Verification items for the finished model (mm, model axes). A direction names the side the tool comes from. Coordinates: 2 decimals unless noted, no trailing zeros. Write each loop counter-clockwise with the first axis right and the second up, starting at its lowest first coordinate (ties: lowest second). Pieces come first, ordered by that corner, then holes. Notation, with made-up numbers: (0.5, -18) -> (57.5, -18) arc R9 ccw to (57.5, -8) -> close; hole circle Ø9 at (-3, 40.5). An arc over 180 degrees is marked (long way). Answer in a Markdown table with one row per item.
```python
from build123d import *

# Parameters (mm, degrees)
SKETCH1_R           = 11
BOSS_EXTRUDE1_DEPTH = 5
BOSS_EXTRUDE2_START = -4
BOSS_EXTRUDE2_DEPTH = 2.5


with BuildPart() as part:
    # Sketch1 → Boss-Extrude1 (new body)
    with BuildSketch(Plane.XY):
        with BuildLine():
            ThreePointArc((4, -41.6), (7.535533906, -43.064466094), (9, -46.6))
            Line((9, -46.6), (9, -61.492137976))
            ThreePointArc((9, -61.492137976), (20.215230476, -65.413125036), (26.544375, -75.467848491))
            ThreePointArc((26.544375, -75.467848491), (30.614674589, -73.910362601), (34.594119865, -72.133534994))
            ThreePointArc((34.594119865, -72.133534994), (31.959737739, -60.548390845), (37.117546722, -49.845468783))
            Line((37.117546722, -49.845468783), (26.587214973, -39.315137034))
            ThreePointArc((26.587214973, -39.315137034), (25.122748879, -35.779603128), (26.587214973, -32.244069222))
            Line((26.587214973, -32.244069222), (32.244069222, -26.587214973))
            ThreePointArc((32.244069222, -26.587214973), (35.779603128, -25.122748879), (39.315137034, -26.587214973))
            Line((39.315137034, -26.587214973), (49.845468783, -37.117546722))
            ThreePointArc((49.845468783, -37.117546722), (60.548390845, -31.959737739), (72.133534994, -34.594119865))
            ThreePointArc((72.133534994, -34.594119865), (73.910362601, -30.614674589), (75.467848491, -26.544375))
            ThreePointArc((75.467848491, -26.544375), (65.413125036, -20.215230476), (61.492137976, -9))
            Line((61.492137976, -9), (46.6, -9))
            ThreePointArc((46.6, -9), (43.064466094, -7.535533906), (41.6, -4))
            Line((41.6, -4), (41.6, 4))
            ThreePointArc((41.6, 4), (43.064466094, 7.535533906), (46.6, 9))
            Line((46.6, 9), (61.492137976, 9))
            ThreePointArc((61.492137976, 9), (65.413125036, 20.215230476), (75.467848491, 26.544375))
            ThreePointArc((75.467848491, 26.544375), (73.910362601, 30.614674589), (72.133534994, 34.594119865))
            ThreePointArc((72.133534994, 34.594119865), (60.548390845, 31.959737739), (49.845468783, 37.117546722))
            Line((49.845468783, 37.117546722), (39.315137034, 26.587214973))
            ThreePointArc((39.315137034, 26.587214973), (35.779603128, 25.122748879), (32.244069222, 26.587214973))
            Line((32.244069222, 26.587214973), (26.587214973, 32.244069222))
            ThreePointArc((26.587214973, 32.244069222), (25.122748879, 35.779603128), (26.587214973, 39.315137034))
            Line((26.587214973, 39.315137034), (37.117546722, 49.845468783))
            ThreePointArc((37.117546722, 49.845468783), (31.959737739, 60.548390845), (34.594119865, 72.133534994))
            ThreePointArc((34.594119865, 72.133534994), (30.614674589, 73.910362601), (26.544375, 75.467848491))
            ThreePointArc((26.544375, 75.467848491), (20.215230476, 65.413125036), (9, 61.492137976))
            Line((9, 61.492137976), (9, 46.6))
            ThreePointArc((9, 46.6), (7.535533906, 43.064466094), (4, 41.6))
            Line((4, 41.6), (-4, 41.6))
            ThreePointArc((-4, 41.6), (-7.535533906, 43.064466094), (-9, 46.6))
            Line((-9, 46.6), (-9, 61.492137976))
            ThreePointArc((-9, 61.492137976), (-20.215230476, 65.413125036), (-26.544375, 75.467848491))
            ThreePointArc((-26.544375, 75.467848491), (-30.614674589, 73.910362601), (-34.594119865, 72.133534994))
            ThreePointArc((-34.594119865, 72.133534994), (-31.959737739, 60.548390845), (-37.117546722, 49.845468783))
            Line((-37.117546722, 49.845468783), (-26.587214973, 39.315137034))
            ThreePointArc((-26.587214973, 39.315137034), (-25.122748879, 35.779603128), (-26.587214973, 32.244069222))
            Line((-26.587214973, 32.244069222), (-32.244069222, 26.587214973))
            ThreePointArc((-32.244069222, 26.587214973), (-35.779603128, 25.122748879), (-39.315137034, 26.587214973))
            Line((-39.315137034, 26.587214973), (-49.845468783, 37.117546722))
            ThreePointArc((-49.845468783, 37.117546722), (-60.548390845, 31.959737739), (-72.133534994, 34.594119865))
            ThreePointArc((-72.133534994, 34.594119865), (-73.910362601, 30.614674589), (-75.467848491, 26.544375))
            ThreePointArc((-75.467848491, 26.544375), (-65.413125036, 20.215230476), (-61.492137976, 9))
            Line((-61.492137976, 9), (-46.6, 9))
            ThreePointArc((-46.6, 9), (-43.064466094, 7.535533906), (-41.6, 4))
            Line((-41.6, 4), (-41.6, -4))
            ThreePointArc((-41.6, -4), (-43.064466094, -7.535533906), (-46.6, -9))
            Line((-46.6, -9), (-61.492137976, -9))
            ThreePointArc((-61.492137976, -9), (-65.413125036, -20.215230476), (-75.467848491, -26.544375))
            ThreePointArc((-75.467848491, -26.544375), (-73.910362601, -30.614674589), (-72.133534994, -34.594119865))
            ThreePointArc((-72.133534994, -34.594119865), (-60.548390845, -31.959737739), (-49.845468783, -37.117546722))
            Line((-49.845468783, -37.117546722), (-39.315137034, -26.587214973))
            ThreePointArc((-39.315137034, -26.587214973), (-35.779603128, -25.122748879), (-32.244069222, -26.587214973))
            Line((-32.244069222, -26.587214973), (-26.587214973, -32.244069222))
            ThreePointArc((-26.587214973, -32.244069222), (-25.122748879, -35.779603128), (-26.587214973, -39.315137034))
            Line((-26.587214973, -39.315137034), (-37.117546722, -49.845468783))
            ThreePointArc((-37.117546722, -49.845468783), (-31.959737739, -60.548390845), (-34.594119865, -72.133534994))
            ThreePointArc((-34.594119865, -72.133534994), (-30.614674589, -73.910362601), (-26.544375, -75.467848491))
            ThreePointArc((-26.544375, -75.467848491), (-20.215230476, -65.413125036), (-9, -61.492137976))
            Line((-9, -61.492137976), (-9, -46.6))
            ThreePointArc((-9, -46.6), (-7.535533906, -43.064466094), (-4, -41.6))
            Line((-4, -41.6), (4, -41.6))
        make_face()
        Circle(SKETCH1_R, mode=Mode.SUBTRACT)
    extrude(amount=BOSS_EXTRUDE1_DEPTH)

    # Sketch2 → Boss-Extrude2 (add)
    with BuildSketch(Plane.XY.offset(5).offset(BOSS_EXTRUDE2_START)):
        with BuildLine():
            ThreePointArc((-37.117546722, 49.845468783), (-31.959737739, 60.548390845), (-34.594119865, 72.133534994))
            ThreePointArc((-34.594119865, 72.133534994), (-42.489529555, 67.783772971), (-49.845468783, 62.573390845))
            Line((-49.845468783, 62.573390845), (-37.117546722, 49.845468783))
        make_face()
        with BuildLine():
            Line((-49.845468783, 37.117546722), (-62.573390845, 49.845468783))
            ThreePointArc((-62.573390845, 49.845468783), (-67.783772971, 42.489529555), (-72.133534994, 34.594119865))
            ThreePointArc((-72.133534994, 34.594119865), (-60.548390845, 31.959737739), (-49.845468783, 37.117546722))
        make_face()
        with BuildLine():
            Line((-9, 61.492137976), (-9, 79.492137976))
            ThreePointArc((-9, 79.492137976), (-17.885731045, 77.975), (-26.544375, 75.467848491))
            ThreePointArc((-26.544375, 75.467848491), (-20.215230476, 65.413125036), (-9, 61.492137976))
        make_face()
        with BuildLine():
            ThreePointArc((9, 61.492137976), (20.215230476, 65.413125036), (26.544375, 75.467848491))
            ThreePointArc((26.544375, 75.467848491), (17.885731045, 77.975), (9, 79.492137976))
            Line((9, 79.492137976), (9, 61.492137976))
        make_face()
        with BuildLine():
            Line((37.117546722, 49.845468783), (49.845468783, 62.573390845))
            ThreePointArc((49.845468783, 62.573390845), (42.489529555, 67.783772971), (34.594119865, 72.133534994))
            ThreePointArc((34.594119865, 72.133534994), (31.959737739, 60.548390845), (37.117546722, 49.845468783))
        make_face()
        with BuildLine():
            ThreePointArc((49.845468783, 37.117546722), (60.548390845, 31.959737739), (72.133534994, 34.594119865))
            ThreePointArc((72.133534994, 34.594119865), (67.783772971, 42.489529555), (62.573390845, 49.845468783))
            Line((62.573390845, 49.845468783), (49.845468783, 37.117546722))
        make_face()
        with BuildLine():
            Line((61.492137976, 9), (79.492137976, 9))
            ThreePointArc((79.492137976, 9), (77.975, 17.885731045), (75.467848491, 26.544375))
            ThreePointArc((75.467848491, 26.544375), (65.413125036, 20.215230476), (61.492137976, 9))
        make_face()
        with BuildLine():
            Line((79.492137976, -9), (61.492137976, -9))
            ThreePointArc((61.492137976, -9), (65.413125036, -20.215230476), (75.467848491, -26.544375))
            ThreePointArc((75.467848491, -26.544375), (77.975, -17.885731045), (79.492137976, -9))
        make_face()
        with BuildLine():
            ThreePointArc((62.573390845, -49.845468783), (67.783772971, -42.489529555), (72.133534994, -34.594119865))
            ThreePointArc((72.133534994, -34.594119865), (60.548390845, -31.959737739), (49.845468783, -37.117546722))
            Line((49.845468783, -37.117546722), (62.573390845, -49.845468783))
        make_face()
        with BuildLine():
            ThreePointArc((34.594119865, -72.133534994), (42.489529555, -67.783772971), (49.845468783, -62.573390845))
            Line((49.845468783, -62.573390845), (37.117546722, -49.845468783))
            ThreePointArc((37.117546722, -49.845468783), (31.959737739, -60.548390845), (34.594119865, -72.133534994))
        make_face()
        with BuildLine():
            ThreePointArc((9, -79.492137976), (17.885731045, -77.975), (26.544375, -75.467848491))
            ThreePointArc((26.544375, -75.467848491), (20.215230476, -65.413125036), (9, -61.492137976))
            Line((9, -61.492137976), (9, -79.492137976))
        make_face()
        with BuildLine():
            ThreePointArc((-26.544375, -75.467848491), (-17.885731045, -77.975), (-9, -79.492137976))
            Line((-9, -79.492137976), (-9, -61.492137976))
            ThreePointArc((-9, -61.492137976), (-20.215230476, -65.413125036), (-26.544375, -75.467848491))
        make_face()
        with BuildLine():
            ThreePointArc((-49.845468783, -62.573390845), (-42.489529555, -67.783772971), (-34.594119865, -72.133534994))
            ThreePointArc((-34.594119865, -72.133534994), (-31.959737739, -60.548390845), (-37.117546722, -49.845468783))
            Line((-37.117546722, -49.845468783), (-49.845468783, -62.573390845))
        make_face()
        with BuildLine():
            ThreePointArc((-72.133534994, -34.594119865), (-67.783772971, -42.489529555), (-62.573390845, -49.845468783))
            Line((-62.573390845, -49.845468783), (-49.845468783, -37.117546722))
            ThreePointArc((-49.845468783, -37.117546722), (-60.548390845, -31.959737739), (-72.133534994, -34.594119865))
        make_face()
        with BuildLine():
            ThreePointArc((-79.492137976, -9), (-77.975, -17.885731045), (-75.467848491, -26.544375))
            ThreePointArc((-75.467848491, -26.544375), (-65.413125036, -20.215230476), (-61.492137976, -9))
            Line((-61.492137976, -9), (-79.492137976, -9))
        make_face()
        with BuildLine():
            ThreePointArc((-75.467848491, 26.544375), (-77.975, 17.885731045), (-79.492137976, 9))
            Line((-79.492137976, 9), (-61.492137976, 9))
            ThreePointArc((-61.492137976, 9), (-65.413125036, 20.215230476), (-75.467848491, 26.544375))
        make_face()
    extrude(amount=BOSS_EXTRUDE2_DEPTH)


solid = part.part
```
1. Sectioned sample at D-D, the plane x = 69.5. Record the cut outline in (y, z).
Findings below:
| item | result |
|---|---|
| outline | (-39.62, 1) -> (-33.23, 1) -> (-33.23, 0) -> (-23.97, 0) -> (-23.97, 1) -> (-9, 1) -> (-9, 3.5) -> (-23.97, 3.5) -> (-23.97, 5) -> (-33.23, 5) -> (-33.23, 3.5) -> (-39.62, 3.5) -> close; (9, 1) -> (23.97, 1) -> (23.97, 0) -> (33.23, 0) -> (33.23, 1) -> (39.62, 1) -> (39.62, 3.5) -> (33.23, 3.5) -> (33.23, 5) -> (23.97, 5) -> (23.97, 3.5) -> (9, 3.5) -> close |
2. Access from +Z, -Z, +X, -X, +Y, -Y to the whole of each face (thin tool, end or side, straight path). Record for faces 4 (the face through (-20.082, 65.308, 0.493)), 5 (the face through (-71, 16, 3.5)), 6 (the face through (31.98, 60.38, 4.24)), 7 (the face through (31.94, -60.72, 0.49)).
Findings below:
| item | result |
|---|---|
| face 4 | -Z, +Y |
| face 5 | +Z, -X |
| face 6 | +Z, +X |
| face 7 | -Z, +X |
3. Sectioned sample at A-A, the plane y = 0. Record the cut outline in (x, z).
Findings below:
| item | result |
|---|---|
| outline | (-41.6, 0) -> (-11, 0) -> (-11, 5) -> (-41.6, 5) -> close; (11, 0) -> (41.6, 0) -> (41.6, 5) -> (11, 5) -> close |
4. Material ranges on probe 1 along X at (y, z) = (-40.5, 2.65); probe 2 along X at (y, z) = (49, 2.3); probe 3 along X at (y, z) = (71.5, 3.9), recorded low to high. Write a range as from..to.
Findings below:
| item | result |
|---|---|
| probe 1 | x = -68.99..-53.23, -27.77..27.77, 53.23..68.99 |
| probe 2 | x = -63.24..-61.73, -36.27..-9, 9..36.27, 61.73..63.24 |
| probe 3 | x = -34.21..-25.13, 25.13..34.21 |
5. Release check for a two-part mould opening along X. For faces 1 (the face through (-31.94, 60.72, 4.24)), 2 (the face through (9, -59, 2)), 3 (the face through (65.308, 20.082, 0.493)) record: released by +X, released by -X, zero draft, split by the parting line, or undercut.
Findings below:
| item | result |
|---|---|
| face 1 | released by -X |
| face 2 | undercut |
| face 3 | released by +X |
6. Sectioned sample at C-C, the plane y = -44.5. Record the cut outline in (x, z), and give its area (3 significant figures).
Findings below:
| item | result |
|---|---|
| outline | (-66.48, 1) -> (-57.23, 1) -> (-57.23, 3.5) -> (-66.48, 3.5) -> close; (-31.77, 0) -> (-8.54, 0) -> (-8.54, 5) -> (-31.77, 5) -> close; (8.54, 0) -> (31.77, 0) -> (31.77, 5) -> (8.54, 5) -> close; (57.23, 1) -> (66.48, 1) -> (66.48, 3.5) -> (57.23, 3.5) -> close |
| area | 279 mm² |
7. Go/stop test with flat-tipped pins: pin 1 (1 mm diameter, centred on x = 1, z = 2.5, fed in from +Y); pin 2 (1.5 mm diameter, centred on y = 60.5, z = 2, fed in from +X); pin 3 (14 mm diameter, centred on x = -70, y = 22, fed in from -Z); pin 4 (1 mm diameter, centred on y = -61, z = 3, fed in from +X). Record where each tip stops, or that it passes through.
Findings below:
| item | result |
|---|---|
| pin 1 | stops at y = 41.6 |
| pin 2 | stops at x = 48.52 |
| pin 3 | stops at z = 0 |
| pin 4 | stops at x = 48.77 |
